```python
from build123d import *

# Parameters (mm, degrees)
F0_W     = 19.05
F0_H     = 25.4
F1_DEPTH = 25.4
F3_DEPTH = 38.1
F4_DEPTH = 25.4


with BuildPart() as f1:
    # F0 (on Front) → F1 (new body)
    with BuildSketch(Plane.XZ):
        with Locations((9.525, 12.7)):
            Rectangle(F0_W, F0_H)
    extrude(amount=-F1_DEPTH)

    # F2 (on Right) → F3 (join)
    with BuildSketch(Plane.YZ):
        Polygon((0, 25.4), (0, 0), (25.4, 0), (25.4, 25.4), (19.05, 25.4), (19.05, 5.828295), (6.35, 5.828295), (6.35, 25.4), align=None)
    extrude(amount=F3_DEPTH)

    # F0 (on Front) → F4 (join)
    with BuildSketch(Plane.XZ):
        Polygon((19.05, 25.4), (19.05, 0), (38.1, 0), align=None)
    extrude(amount=-F4_DEPTH)


solid = f1.part
```
Geometry check sheet. Reference: the model listing, model coordinates, mm. A direction names the side the tool comes from. Round coordinates to 2 decimals unless told otherwise and drop trailing zeros. Loops run counter-clockwise (first coordinate to the right, second up) from the corner with the lowest first, then second, coordinate; pieces in that order, holes last. Notation, with made-up numbers: (2.25, 64.25) - (49.25, 64.25) arc R14 ccw to (49.25, 79.25) - close; hole circle Ø7 at (-27, 24). An arc over 180 degrees is marked (long way). Use a Markdown table: item, result.
Q1. Material ranges on line 1 (Y direction, x = 28.5, z = 16); line 2 (Z direction, x = 35.5, y = 15.75); line 3 (X direction, y = 14.5, z = 13), recorded low to high.
Solutions:
| item | result |
|---|---|
| line 1 | y = 0 to 6.35, 19.05 to 25.4 |
| line 2 | z = 0 to 5.83 |
| line 3 | x = 0 to 28.35 |
Q2. Access from +Z, -Z, +X, -X, +Y, -Y to the whole of each face (thin tool, end or side, straight path). Record for faces 1 (the flat face through (0, 13, 13)), 2 (the flat face through (31, 19.05, 18)).
Solutions:
| item | result |
|---|---|
| face 1 | +Z, -Z, -X, +Y, -Y |
| face 2 | +Z, +X |
Q3. Go/stop test with a flat-tipped pin: P1, Ø5, axis at x = 36, y = 11, coming from the +Z side. Record where the tip stops, or that it passes through.
Solutions:
| item | result |
|---|---|
| P1 | stops at z = 6.13 |
Q4. Cross-section at C-C on y = 11.5. Record the cut outline in (x, z).
Solutions:
| item | result |
|---|---|
| outline | (0, 0) - (38.1, 0) - (38.1, 5.83) - (33.73, 5.83) - (19.05, 25.4) - (0, 25.4) - close |
Q5. Cross-section at A-A on x = 22.5. Record the cut outline in (y, z).
Solutions:
| item | result |
|---|---|
| outline | (0, 0) - (25.4, 0) - (25.4, 25.4) - (19.05, 25.4) - (19.05, 20.8) - (6.35, 20.8) - (6.35, 25.4) - (0, 25.4) - close |
Q6. Cross-section at B-B on z = 19. Record the cut outline in (x, y), plus the area to 3 significant figures.
Solutions:
| item | result |
|---|---|
| outline | (0, 0) - (38.1, 0) - (38.1, 6.35) - (23.85, 6.35) - (23.85, 19.05) - (38.1, 19.05) - (38.1, 25.4) - (0, 25.4) - close |
| area | 787 mm2 |
Q7. Draft check along Y on faces 3 (the flat face through (15, 13, 25.4)), 4 (the flat face through (19, 0, 13)), 5 (the flat face through (36, 13, 5.828)), 6 (the flat face through (19, 25.4, 13)). Enter one of: released by +Y, released by -Y, zero draft, split by the parting line, or undercut.
Solutions:
| item | result |
|---|---|
| face 3 | zero draft |
| face 4 | released by -Y |
| face 5 | undercut |
| face 6 | released by +Y |
